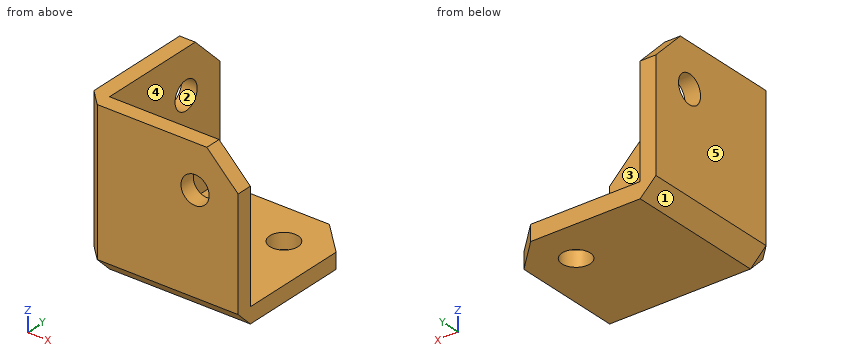
from build123d import *

# Parameters (mm, degrees)
SKETCH2_W           = 25.4
SKETCH2_H           = 25.4
BOSS_EXTRUDE2_DEPTH = 25.4
SKETCH3_W           = 22.86
SKETCH3_H           = 22.86
CUT_EXTRUDE1_DEPTH  = 22.86
SKETCH4_R           = 2.286
CUT_EXTRUDE3_DEPTH  = 2.54
SKETCH5_R           = 2.286
CUT_EXTRUDE4_DEPTH  = 2.54
SKETCH6_R           = 2.286
CUT_EXTRUDE5_DEPTH  = 2.54
CHAMFER1_SIZE       = 5.08
CHAMFER2_SIZE       = 2.54


with BuildPart() as part:
    # Sketch2 → Boss-Extrude2 (new body)
    with BuildSketch(Plane.XY):
        with Locations((12.7, 12.7)):
            Rectangle(SKETCH2_W, SKETCH2_H)
    extrude(amount=BOSS_EXTRUDE2_DEPTH)

    # Sketch3 → Cut-Extrude1 (cut)
    with BuildSketch(Plane.XY.offset(25.4)):
        with Locations((13.97, 13.97)):
            Rectangle(SKETCH3_W, SKETCH3_H)
    extrude(amount=-CUT_EXTRUDE1_DEPTH, mode=Mode.SUBTRACT)

    # Sketch4 → Cut-Extrude3 (cut)
    with BuildSketch(Plane.XY.offset(2.54)):
        with Locations((18.415, 18.415)):
            Circle(SKETCH4_R)
    extrude(amount=-CUT_EXTRUDE3_DEPTH, mode=Mode.SUBTRACT)

    # Sketch5 → Cut-Extrude4 (cut)
    with BuildSketch(Plane(origin=(2.54, 0, 0), x_dir=(0, 0, -1), z_dir=(1, 0, 0))):
        with Locations((-18.415, 18.415)):
            Circle(SKETCH5_R)
    extrude(amount=-CUT_EXTRUDE4_DEPTH, mode=Mode.SUBTRACT)

    # Sketch6 → Cut-Extrude5 (cut)
    with BuildSketch(Plane(origin=(0, 2.54, 0), x_dir=(1, 0, 0), z_dir=(0, 1, 0))):
        with Locations((18.415, -18.415)):
            Circle(SKETCH6_R)
    extrude(amount=-CUT_EXTRUDE5_DEPTH, mode=Mode.SUBTRACT)

    # Chamfer1
    chamfer1_edges = [part.edges().sort_by_distance(p)[0] for p in [
        (25.4, 1.27, 25.4),
        (1.27, 25.4, 25.4),
        (25.4, 25.4, 1.27),
    ]]
    chamfer(chamfer1_edges, length=CHAMFER1_SIZE)

    # Chamfer2
    chamfer2_edges = [part.edges().sort_by_distance(p)[0] for p in [
        (12.7, 0, 0),
        (0, 12.7, 0),
        (0, 0, 12.7),
    ]]
    chamfer(chamfer2_edges, length=CHAMFER2_SIZE)


solid = part.part
Design review of the part built by this model. Coordinates are the model's own, in mm. Face numbers are marked on the shaded views. A direction names the side the tool comes from. Coordinates: 2 decimals unless noted, no trailing zeros. Write each loop counter-clockwise with the first axis right and the second up, starting at its lowest first coordinate (ties: lowest second). Pieces come first, ordered by that corner, then holes. Notation, with made-up numbers: (58.25, -19.75) -> (64.25, -19.75) arc R20 ccw to (64.25, 4.25) -> close; hole circle Ø8 at (-2, 70.25). An arc over 180 degrees is marked (long way). Write each question's results on one line, items separated by ' | '. Start each with the question number.
(1) Tool access review of the marked faces 4 and 5: name each direction out of +Z, -Z, +X, -X, +Y, -Y from which nothing blocks a thin tool from reaching the whole face with its end or side.
(2) For line 1 along Z through (x, y) = (4.5, 5.25), list the stretches that pass through material, from the lowest coordinate up. Write a range as from..to.
(3) Take a section at A-A on z = 15.25. Write out the cut boundary in (x, y).
(4) Take a section at D-D on z = 1.75. Write out the cut boundary in (x, y) (3 decimals).
(5) The part is to be moulded in two halves that separate along Z. For the marked faces 1, 2 and 3, say which applies: pulls with the +Z half, pulls with the -Z half, needs draft (parallel to the pull), parting line crosses it, or undercut.
(6) Take a section at C-C on z = 18. Write out the cut boundary in (x, y).
(7) Clearance check with flat-ended pins moving along their axes: P1, Ø5, axis at x = 8.5, z = 13.5, coming from the +Y side; P2, Ø5.5, axis at x = 18.415, y = 18.415, coming from the +Z side; P3, Ø2, axis at y = 17.5, z = 20.5, coming from the -X side; P4, Ø2, axis at y = 6, z = 6, coming from the +X side. State where each tip first meets the part, or that it passes through.
Results found:
1) face 4: +Z, +X, +Y | face 5: +Z, -Z, -X, +Y, -Y
2) line 1: z = 0..2.54
3) outline: (0, 2.54) -> (2.54, 0) -> (25.4, 0) -> (25.4, 2.54) -> (2.54, 2.54) -> (2.54, 25.4) -> (0, 25.4) -> close
4) outline: (0.79, 2.54) -> (2.54, 0.79) -> (25.4, 0.79) -> (25.4, 20.32) -> (20.32, 25.4) -> (0.79, 25.4) -> close; hole circle Ø4.572 at (18.415, 18.415)
5) face 1: pulls with the -Z half | face 2: undercut | face 3: needs draft
6) outline: (0, 2.54) -> (2.54, 0) -> (16.17, 0) -> (16.17, 2.54) -> (2.54, 2.54) -> (2.54, 16.17) -> (0, 16.17) -> close; (0, 20.66) -> (2.54, 20.66) -> (2.54, 25.4) -> (0, 25.4) -> close; (20.66, 0) -> (25.4, 0) -> (25.4, 2.54) -> (20.66, 2.54) -> close
7) P1: stops at y = 2.54 | P2: stops at z = 2.54 | P3: stops at x = 0 | P4: stops at x = 2.54
